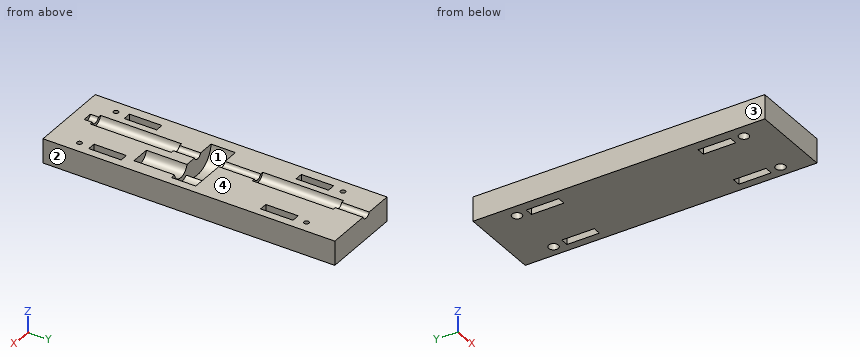
```python
from build123d import *

# Parameters (mm, degrees)
SKETCH006_R     = 3.15
PAD002_DEPTH    = 190
SKETCH011_R     = 5
PAD007_DEPTH    = 50
SKETCH010_R     = 5
PAD006_DEPTH    = 50
SKETCH008_R     = 13
PAD004_DEPTH    = 15
SKETCH009_R     = 9
PAD005_DEPTH    = 15
SKETCH013_R     = 6
PAD008_DEPTH    = 26
BOX001_W        = 50
BOX001_H        = 180
BOX001_DEPTH    = 15
SKETCH015_R     = 1.5
POCKET001_DEPTH = 389.834296
SKETCH016_R     = 1.5
POCKET002_DEPTH = 389.834296
SKETCH017_R     = 3
POCKET003_DEPTH = 5
SKETCH018_R     = 3
POCKET004_DEPTH = 5
SKETCH022_W     = 5
SKETCH022_H     = 20
POCKET008_DEPTH = 389.834296
SKETCH023_W     = 5
SKETCH023_H     = 20
POCKET009_DEPTH = 389.834296


with BuildPart() as pad002:
    # Sketch006 → Pad002 (new body)
    with BuildSketch(Plane.XZ.offset(80)):
        Circle(SKETCH006_R)
    extrude(amount=-PAD002_DEPTH)


with BuildPart() as pad007:
    # Sketch011 → Pad007 (new body)
    with BuildSketch(Plane.XZ.offset(-75)):
        Circle(SKETCH011_R)
    extrude(amount=PAD007_DEPTH)


with BuildPart() as scassi_perno:
    # Sketch010 → Pad006 (new body)
    with BuildSketch(Plane.XZ.offset(25)):
        Circle(SKETCH010_R)
    extrude(amount=PAD006_DEPTH)

    # Fusion002: union Pad007
    add(pad007.part)


with BuildPart() as scasso_ruota_dentata:
    # Sketch008 → Pad004 (new body)
    with BuildSketch(Plane.XZ.offset(-3)):
        Circle(SKETCH008_R)
    extrude(amount=PAD004_DEPTH)


with BuildPart() as obj1:
    # Sketch009 → Pad005 (new body)
    with BuildSketch(Plane.XZ.offset(-3)):
        with Locations((15.997087, 9e-06)):
            Circle(SKETCH009_R)
    extrude(amount=PAD005_DEPTH)

    # Fusion001: union scasso_ruota_dentata
    add(scasso_ruota_dentata.part)


with BuildPart() as fusion:
    # Sketch013 → Pad008 (new body)
    with BuildSketch(Plane.XZ.offset(11)):
        with Locations((16.059561, 9e-06)):
            Circle(SKETCH013_R)
    extrude(amount=PAD008_DEPTH)

    # Fusion005: union scassi_perno, obj1
    add(scassi_perno.part)
    add(obj1.part)

    # Fusion: union Pad002
    add(pad002.part)


with BuildPart() as obj2:
    # Box001 → Box001 (new body)
    with BuildSketch(Plane(origin=(-20, -88, -16), x_dir=(1, 0, 0), z_dir=(0, 0, 1))):
        with Locations((25, 90)):
            Rectangle(BOX001_W, BOX001_H)
    extrude(amount=BOX001_DEPTH)

    # Cut001: cut Fusion
    add(fusion.part, mode=Mode.SUBTRACT)

    # Sketch015 → Pocket001 (cut, through all)
    with BuildSketch(Plane(origin=(0, 0, -16), x_dir=(1, 0, 0), z_dir=(0, 0, -1))):
        with Locations((23, 70)):
            Circle(SKETCH015_R)
    pocket001 = extrude(amount=-POCKET001_DEPTH, mode=Mode.SUBTRACT)

    # Mirrored: Pocket001 across Sketch015 H_Axis
    add(pocket001.mirror(Plane(origin=(0, 0, -16), x_dir=(0, 0, -1), z_dir=(0, -1, 0))), mode=Mode.SUBTRACT)

    # Sketch016 → Pocket002 (cut, through all)
    with BuildSketch(Plane(origin=(0, 0, -16), x_dir=(1, 0, 0), z_dir=(0, 0, -1))):
        with Locations((-12, 70)):
            Circle(SKETCH016_R)
    pocket002 = extrude(amount=-POCKET002_DEPTH, mode=Mode.SUBTRACT)

    # Mirrored001: Pocket002 across Sketch016 H_Axis
    add(pocket002.mirror(Plane(origin=(0, 0, -16), x_dir=(0, 0, -1), z_dir=(0, -1, 0))), mode=Mode.SUBTRACT)

    # Sketch017 → Pocket003 (cut)
    with BuildSketch(Plane(origin=(0, 0, -16), x_dir=(1, 0, 0), z_dir=(0, 0, -1))):
        with Locations((23, 70)):
            Circle(SKETCH017_R)
    pocket003 = extrude(amount=-POCKET003_DEPTH, mode=Mode.SUBTRACT)

    # Mirrored002: Pocket003 across Sketch017 H_Axis
    add(pocket003.mirror(Plane(origin=(0, 0, -16), x_dir=(0, 0, -1), z_dir=(0, -1, 0))), mode=Mode.SUBTRACT)

    # Sketch018 → Pocket004 (cut)
    with BuildSketch(Plane(origin=(0, 0, -16), x_dir=(1, 0, 0), z_dir=(0, 0, -1))):
        with Locations((-12, 70)):
            Circle(SKETCH018_R)
    pocket004 = extrude(amount=-POCKET004_DEPTH, mode=Mode.SUBTRACT)

    # Mirrored003: Pocket004 across Sketch018 H_Axis
    add(pocket004.mirror(Plane(origin=(0, 0, -16), x_dir=(0, 0, -1), z_dir=(0, -1, 0))), mode=Mode.SUBTRACT)

    # Sketch022 → Pocket008 (cut, through all)
    with BuildSketch(Plane(origin=(0, 0, -16), x_dir=(1, 0, 0), z_dir=(0, 0, -1))):
        with Locations((22.5, 53)):
            Rectangle(SKETCH022_W, SKETCH022_H)
    pocket008 = extrude(amount=-POCKET008_DEPTH, mode=Mode.SUBTRACT)

    # Mirrored006: Pocket008 across Sketch022 H_Axis
    add(pocket008.mirror(Plane(origin=(0, 0, -16), x_dir=(0, 0, -1), z_dir=(0, -1, 0))), mode=Mode.SUBTRACT)

    # Sketch023 → Pocket009 (cut, through all)
    with BuildSketch(Plane(origin=(0, 0, -16), x_dir=(1, 0, 0), z_dir=(0, 0, -1))):
        with Locations((-11.5, 53)):
            Rectangle(SKETCH023_W, SKETCH023_H)
    pocket009 = extrude(amount=-POCKET009_DEPTH, mode=Mode.SUBTRACT)

    # Mirrored007: Pocket009 across Sketch023 H_Axis
    add(pocket009.mirror(Plane(origin=(0, 0, -16), x_dir=(0, 0, -1), z_dir=(0, -1, 0))), mode=Mode.SUBTRACT)


solid = obj2.part
```
Here's how the part is built. I have some questions about the finished solid (model axes, mm). Face numbers are marked on the shaded views. Round coordinates to 2 decimals unless told otherwise and drop trailing zeros. Order: outer loops, then holes, each group sorted by start corner. A loop starts at its lowest first (then second) coordinate and runs counter-clockwise, first axis right, second up. Notation, with made-up numbers: (31, 46.25) -> (87, 46.25) arc R13 cw to (87, 69.25) -> close; hole circle Ø11 at (5, -28.5). An arc over 180 degrees is marked (long way). Use a Markdown table: item, result. Add a question column.
(1) For pin 1 Ø3.5 at (x, y) = (-12, 70) entering from -Z; pin 2 Ø1.7 at (x, z) = (-1, -2) entering from +Y, each with a flat end and sliding along its axis, tell me the tip position at first contact or that it passes through.
(2) Suppose I cut it at A-A, the plane y = -61. Please give me the cut outline in (x, z).
(3) Suppose I cut it at C-C, the plane y = -14.5. Please give me the cut outline in (x, z), and give its area (3 significant figures).
(4) If we mould it in two halves opening along X, with no side actions, what happens to the marked faces 1, 2, 3 and 4? For each: released by +X, released by -X, zero draft, split by the parting line, or undercut.
(5) Suppose I cut it at D-D, the plane x = 13. Please give me the cut outline in (y, z), and give its area (3 significant figures).
(6) Suppose I cut it at B-B, the plane x = 0. Please give me the cut outline in (y, z).
(7) I need wall thicknesses on line 1 along X through (y, z) = (70, -7.5); line 2 along Y through (x, z) = (-12, -13.15); line 3 along X through (y, z) = (70, -14.85). Which ranges of each line are inside material? Lowest first, please.
Verdict:
| question | item | result |
|---|---|---|
| 1 | pin 1 | z = -11 |
| 1 | pin 2 | y = -80 |
| 2 | outline | (-20, -16) -> (-14, -16) -> (-14, -1) -> (-20, -1) -> close; (-9, -16) -> (20, -16) -> (20, -1) -> (4.9, -1) arc R5 cw to (-4.9, -1) -> (-9, -1) -> close; (25, -16) -> (30, -16) -> (30, -1) -> (25, -1) -> close |
| 3 | outline | (-20, -16) -> (30, -16) -> (30, -1) -> (21.98, -1) arc R6 cw to (10.14, -1) -> (2.99, -1) arc R3.15 cw to (-2.99, -1) -> (-20, -1) -> close |
| 3 | area | 696 mm2 |
| 4 | face 1 | undercut |
| 4 | face 2 | released by +X |
| 4 | face 3 | released by -X |
| 4 | face 4 | zero draft |
| 5 | outline | (-88, -16) -> (92, -16) -> (92, -1) -> (3, -1) -> (3, -8.49) -> (-12, -8.49) -> (-12, -5.16) -> (-37, -5.16) -> (-37, -1) -> (-88, -1) -> close |
| 5 | area | 2,480 mm2 |
| 6 | outline | (-88, -16) -> (92, -16) -> (92, -3.15) -> (75, -3.15) -> (75, -5) -> (25, -5) -> (25, -3.15) -> (3, -3.15) -> (3, -13) -> (-12, -13) -> (-12, -3.15) -> (-25, -3.15) -> (-25, -5) -> (-75, -5) -> (-75, -3.15) -> (-80, -3.15) -> (-80, -1) -> (-88, -1) -> close |
| 7 | line 1 | -20 to -13.5, -10.5 to 21.5, 24.5 to 30 |
| 7 | line 2 | -88 to -73, -67 to -63, -43 to 43, 63 to 67, 73 to 92 |
| 7 | line 3 | -20 to -15, -9 to 20, 26 to 30 |
